For this review, take the finished solid that the model builds, in its own axes (mm). Face numbers are marked on the shaded views. A direction names the side the tool comes from. Coordinates: 2 decimals unless noted, no trailing zeros. Order: outer loops, then holes, each group sorted by start corner. A loop starts at its lowest first (then second) coordinate and runs counter-clockwise, first axis right, second up. Notation, with made-up numbers: M -33,-20.75 L -13,-20.75 A16 cw -13,1.25 Z; hole C 80,-8.75 d3. An arc over 180 degrees is marked long. Use CSV: the item, a comma, the result in double quotes.
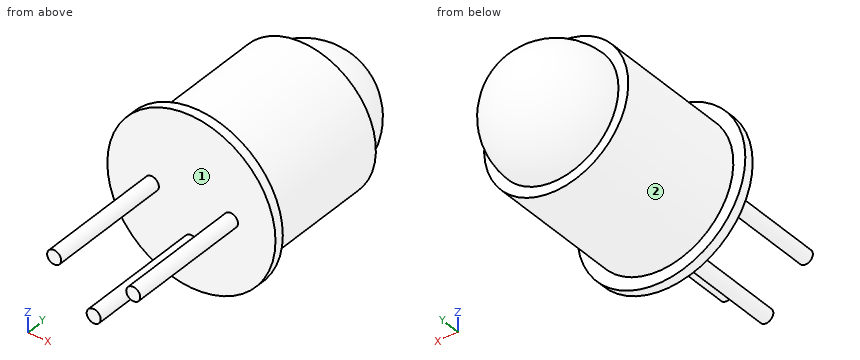
```python
from build123d import *

# Parameters (mm, degrees)
SKETCH_1_R      = 2.315
EXTRUDE_1_DEPTH = 4.3
SKETCH_3_R      = 2.7
EXTRUDE_2_DEPTH = 0.3
SKETCH_5_R      = 0.225
EXTRUDE_3_DEPTH = 4


with BuildPart() as part:
    # 草图1 → 凸台-拉伸1 (new body)
    with BuildSketch(Plane(origin=(0, 0, 0), x_dir=(1, 0, 0), z_dir=(0, 1, 0))):
        with Locations(Location((0, 0, 0), (0, 0, 90))):
            Circle(SKETCH_1_R)
    extrude(amount=EXTRUDE_1_DEPTH)

    # 草图2 → 旋转2 (revolve)
    with BuildSketch(Plane.XY):
        with BuildLine():
            Line((-2, 4.3), (0, 4.3))
            Line((0, 4.3), (0, 6.3))
            ThreePointArc((0, 6.3), (-1.414213562, 5.714213562), (-2, 4.3))
        make_face()
    revolve(axis=Axis((0, 11.522957205, 0), (0, -1, 0)))

    # 草图3 → 凸台-拉伸2 (add)
    with BuildSketch(Plane.XZ):
        with Locations(Location((0, 0, 0), (0, 0, 270))):
            Circle(SKETCH_3_R)
    extrude(amount=EXTRUDE_2_DEPTH)

    # 草图5 → 凸台-拉伸3 (add)
    with BuildSketch(Plane.XZ.offset(0.3)):
        with Locations(Location((-1.27, 0, 0), (0, 0, 270))):
            Circle(SKETCH_5_R)
        with Locations(Location((1.27, 0, 0), (0, 0, 270))):
            Circle(SKETCH_5_R)
        with Locations(Location((0, -1.27, 0), (0, 0, 270))):
            Circle(SKETCH_5_R)
    extrude(amount=EXTRUDE_3_DEPTH)


solid = part.part
```
Item 1: Add section D-D on y = 5.5. State the section outline as (x, z) points.
Solutions:
outline,"C 0,0 d3.2"
Item 2: Add section A-A on z = 0. State the section outline as (x, y) points (3 decimals), and give its area (3 significant figures).
Solutions:
outline,"M -2.7,-0.3 L -1.495,-0.3 L -1.495,-4.3 L -1.045,-4.3 L -1.045,-0.3 L 1.045,-0.3 L 1.045,-4.3 L 1.495,-4.3 L 1.495,-0.3 L 2.7,-0.3 L 2.7,0 L 2.315,0 L 2.315,4.3 L 2,4.3 A2 ccw -2,4.3 L -2.315,4.3 L -2.315,0 L -2.7,0 Z"
area,"31.4 mm^2"
Item 3: Clearance check with flat-ended pins moving along their axes: pin 1 Ø1.5 at (x, z) = (1.5, 0.5) entering from +Y; pin 2 Ø1 at (x, z) = (0, 1.5) entering from +Y; pin 3 Ø3 at (y, z) = (0.5, 2) entering from +X. State where each tip first meets the part, or that it passes through.
Solutions:
pin 1,"y = 6.12"
pin 2,"y = 6.03"
pin 3,"x = 2.64"
Item 4: To check wall thickness, follow line 1 along Y through (x, z) = (-1, 2.25); line 2 along Y through (x, z) = (-0.5, 2); line 3 along X through (y, z) = (1, -0.1). State the ranges of each line that lie inside material, in increasing order. Write a range as [from, to].
Solutions:
line 1,"[-0.3, 0]"
line 2,"[-0.3, 4.3]"
line 3,"[-2.31, 2.31]"
Item 5: Add section B-B on y = -3. State the section outline as (x, z) points (3 decimals), and give its area (3 significant figures).
Solutions:
outline,"C -1.27,0 d0.45; C 0,-1.27 d0.45; C 1.27,0 d0.45"
area,"0.477 mm^2"
Item 6: For the marked faces 1 and 2, list the 3-axis set-ups (+Z, -Z, +X, -X, +Y, -Y) from which the entire face can be reached by the end or side of a thin tool; tool diameter is ignored.
Solutions:
face 1,"-Y"
face 2,"+Y"
Item 7: Add section C-C on x = 0.7. State the section outline as (y, z) points, and give its area (3 significant figures).
Solutions:
outline,"M -0.3,-2.61 L 0,-2.61 L 0,-2.21 L 4.3,-2.21 L 4.3,-1.87 A1.87 ccw 4.3,1.87 L 4.3,2.21 L 0,2.21 L 0,2.61 L -0.3,2.61 Z"
area,"26.1 mm^2"
